Model file for the job. Use its own axes, mm. A direction names the side the tool comes from. Coordinates: 2 decimals unless noted, no trailing zeros. Write each loop counter-clockwise with the first axis right and the second up, starting at its lowest first coordinate (ties: lowest second). Pieces come first, ordered by that corner, then holes.
Q1. Band-saw the part on C-C, the plane z = 5.5. Write the cut outline in (x, y).
Q2. Which spindle directions (+Z, -Z, +X, -X, +Y, -Y) get a long thin tool onto all of the face, cutting with end or side? Do faces 1 (the flat face through (-1, 50, 5)), 2 (the flat face through (-70, -10, 5)). Say none if no direction does.
Q3. Band-saw the part on D-D, the plane y = 0. Write the cut outline in (x, z), plus the area to 3 significant figures.
Q4. Band-saw the part on A-A, the plane y = 33.5. Write the cut outline in (x, z), plus the area to 3 significant figures.
Q5. Band-saw the part on B-B, the plane x = 20. Write the cut outline in (y, z), plus the area to 3 significant figures.
Q6. Drill centre lines: probe 1 along Y at (x, z) = (27.5, 4.25); probe 2 along Y at (x, z) = (66, 8.25); probe 3 along Y at (x, z) = (-65.5, 1.75). Where is each one in solid material? Low to high.
Q7. Pull direction Z, two halves, no side cores. Call faces 3 (the flat face through (-70, 10, 5)), 4 (the flat face through (-1, 1, 10)), 5 (the flat face through (-1, 1, 0)): released by +Z, released by -Z, zero draft, split by the parting line, or undercut.
from build123d import *

# Parameters (mm, degrees)
F0_R     = 3.4
F0_R_2   = 12.5
F1_DEPTH = 10


with BuildPart() as f1:
    # F0 (on Top) → F1 (new body)
    with BuildSketch(Plane.XY):
        with BuildLine():
            ThreePointArc((75, 45), (73.535534, 48.535534), (70, 50))
            Line((70, 50), (-75, 50))
            Line((-75, 50), (-75, 10))
            Line((-75, 10), (-65, 10))
            ThreePointArc((-65, 10), (-55, 0), (-65, -10))
            Line((-65, -10), (-75, -10))
            Line((-75, -10), (-75, -50))
            Line((-75, -50), (70, -50))
            ThreePointArc((70, -50), (73.535534, -48.535534), (75, -45))
            Line((75, -45), (75, 45))
        make_face()
        with Locations((63.891, -33.5)):
            Circle(F0_R, mode=Mode.SUBTRACT)
        with Locations((-15, 0)):
            Circle(F0_R, mode=Mode.SUBTRACT)
        with Locations((27.5, 0)):
            Circle(F0_R_2, mode=Mode.SUBTRACT)
        with Locations((63.891, 33.5)):
            Circle(F0_R, mode=Mode.SUBTRACT)
    extrude(amount=F1_DEPTH)


solid = f1.part
Answer sheet:
1. outline: (-75, -50) - (70, -50) arc R5 ccw to (75, -45) - (75, 45) arc R5 ccw to (70, 50) - (-75, 50) - (-75, 10) - (-65, 10) arc R10 cw to (-65, -10) - (-75, -10) - close; hole circle Ø6.8 at (-15, 0); hole circle Ø25 at (27.5, 0); hole circle Ø6.8 at (63.89, -33.5); hole circle Ø6.8 at (63.89, 33.5)
2. face 1: +Z, -Z, +X, -X, +Y
2. face 2: +Z, -Z, -X
3. outline: (-55, 0) - (-18.4, 0) - (-18.4, 10) - (-55, 10) - close; (-11.6, 0) - (15, 0) - (15, 10) - (-11.6, 10) - close; (40, 0) - (75, 0) - (75, 10) - (40, 10) - close
3. area: 982 mm2
4. outline: (-75, 0) - (60.49, 0) - (60.49, 10) - (-75, 10) - close; (67.29, 0) - (75, 0) - (75, 10) - (67.29, 10) - close
4. area: 1,430 mm2
5. outline: (-50, 0) - (-10, 0) - (-10, 10) - (-50, 10) - close; (10, 0) - (50, 0) - (50, 10) - (10, 10) - close
5. area: 800 mm2
6. probe 1: y = -50 to -12.5, 12.5 to 50
6. probe 2: y = -50 to -36.17, -30.83 to 30.83, 36.17 to 50
6. probe 3: y = -50 to -10, 10 to 50
7. face 3: zero draft
7. face 4: released by +Z
7. face 5: released by -Z
